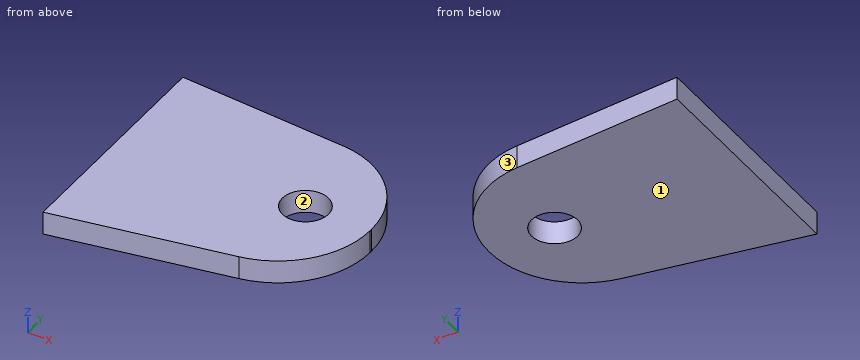
from build123d import *

# Parameters (mm, degrees)
SKETCH1_W                       = 66.08808118
SKETCH1_H                       = 37.717352964
BOSS_EXTRUDE1_DEPTH             = 3.175
F_1_4_0_25_DIAMETER_HOLE1_D     = 6.35
F_1_4_0_25_DIAMETER_HOLE1_DEPTH = 9.268267535
F_1_4_0_25_DIAMETER_HOLE1_TIP   = 1.907732465
CUT_EXTRUDE1_DEPTH              = 43.378010118
FILLET1_R                       = 12.7


with BuildPart() as part:
    # Sketch1 → Boss-Extrude1 (new body)
    with BuildSketch(Plane.XY):
        with Locations((3.763463947, 1.902410347)):
            Rectangle(SKETCH1_W, SKETCH1_H)
    extrude(amount=BOSS_EXTRUDE1_DEPTH)

    # 1/4 (0.25) Diameter Hole1
    with Locations(Plane.XY.offset(3.175)):
        with Locations((-3.439886643, 6.028832829)):
            Hole(F_1_4_0_25_DIAMETER_HOLE1_D / 2, depth=F_1_4_0_25_DIAMETER_HOLE1_DEPTH)
            with Locations((0, 0, -(F_1_4_0_25_DIAMETER_HOLE1_DEPTH + F_1_4_0_25_DIAMETER_HOLE1_TIP / 2))):  # 118° drill point
                Cone(0, F_1_4_0_25_DIAMETER_HOLE1_D / 2, F_1_4_0_25_DIAMETER_HOLE1_TIP, mode=Mode.SUBTRACT)

    # Sketch4 → Cut-Extrude1 (cut, through all)
    with BuildSketch(Plane(origin=(0, 0, 0), x_dir=(-1, 0, 0), z_dir=(0, 0, -1))):
        Polygon((-5.644423357, 17.705545255), (29.280576643, 20.761086829), (-36.807504537, 20.761086829), (-36.807504537, -16.956266135), (29.280576643, -16.956266135), (29.280576643, -11.068161171), (-5.644423357, -4.90994137), align=None)
    extrude(amount=-CUT_EXTRUDE1_DEPTH, mode=Mode.SUBTRACT)

    # Fillet1
    fillet1_edges = [part.edges().sort_by_distance(p)[0] for p in [
        (5.644423357, 17.705545255, 1.5875),
        (5.644423357, -4.90994137, 1.5875),
    ]]
    fillet(fillet1_edges, radius=FILLET1_R)


solid = part.part
Verification items for the finished model (mm, model axes). Face numbers are marked on the shaded views. Give positions to 0.01 mm unless a question says otherwise; leave off trailing zeros. Order: outer loops, then holes, each group sorted by start corner. A loop starts at its lowest first (then second) coordinate and runs counter-clockwise, first axis right, second up. Notation, with made-up numbers: (40, 45.25) -> (92, 45.25) arc R9 cw to (92, 53.25) -> close; hole circle Ø8 at (-13, 82). An arc over 180 degrees is marked (long way). Answer as CSV lines item,"result".
Q1. Sectioned sample at C-C on x = -4. Record the cut outline in (y, z) (3 decimals), plus the area to 3 significant figures.
Solutions:
outline,"(-6.58, 0) -> (2.904, 0) -> (2.904, 3.175) -> (-6.58, 3.175) -> close; (9.154, 0) -> (18.395, 0) -> (18.395, 3.175) -> (9.154, 3.175) -> close"
area,"59.5 mm²"
Q2. Release check for a two-part mould opening along X. For the marked faces 1, 2 and 3 record: +X half, -X half, draft (parallel to the pull), parting line (faces both ways), or undercut.
Solutions:
face 1,"draft"
face 2,"undercut"
face 3,"+X half"
Q3. Scan lines: probe 1 along X at (y, z) = (14, 1.5); probe 2 along Y at (x, z) = (-2, 1); probe 3 along Y at (x, z) = (-4.5, 0.3). Record each from-to range of solid material in increasing order.
Solutions:
probe 1,"x = -29.28 to 2.86"
probe 2,"y = -5.9 to 3.2, 8.86 to 17.72"
probe 3,"y = -6.69 to 3.04, 9.02 to 18.51"
Q4. Sectioned sample at A-A on z = 1.25. Record the cut outline in (x, y) (3 decimals).
Solutions:
outline,"(-29.281, -11.068) -> (-4.85, -6.76) arc R12.7 ccw to (5.644, 5.747) -> (5.644, 6.068) arc R12.7 ccw to (-5.949, 18.72) -> (-29.281, 20.761) -> close; hole circle Ø6.35 at (-3.44, 6.029)"
Q5. Sectioned sample at D-D on x = -24.5. Record the cut outline in (y, z) (3 decimals), plus the area to 3 significant figures.
Solutions:
outline,"(-10.225, 0) -> (20.343, 0) -> (20.343, 3.175) -> (-10.225, 3.175) -> close"
area,"97.1 mm²"
Q6. Sectioned sample at B-B on y = 8. Record the cut outline in (x, z) (3 decimals).
Solutions:
outline,"(-29.281, 0) -> (-5.929, 0) -> (-5.929, 3.175) -> (-29.281, 3.175) -> close; (-0.951, 0) -> (5.497, 0) -> (5.497, 3.175) -> (-0.951, 3.175) -> close"
